Part model, mm, in its own coordinate system. A direction names the side the tool comes from. Round coordinates to 2 decimals unless told otherwise and drop trailing zeros. Loops run counter-clockwise (first coordinate to the right, second up) from the corner with the lowest first, then second, coordinate; pieces in that order, holes last. Notation, with made-up numbers: M 38,-3.75 L 57,-3.75 A21 ccw 57,34.25 Z; hole C 49,78 d6. An arc over 180 degrees is marked long. Write each question's results on one line, items separated by ' | '.
from build123d import *

# Parameters (mm, degrees)
BOSS_EXTRUDE1_DEPTH = 6.35
SKETCH9_R           = 3.175
CUT_EXTRUDE3_DEPTH  = 7.35
CIRPATTERN6_COUNT   = 3
CUT_EXTRUDE4_DEPTH  = 7.35
BOSS_EXTRUDE4_DEPTH = 6.35
CIRPATTERN7_COUNT   = 6


with BuildPart() as part:
    # Sketch1 → Boss-Extrude1 (new body)
    with BuildSketch(Plane(origin=(0, 0, 0), x_dir=(1, 0, 0), z_dir=(0, 1, 0))):
        Polygon((88.9, 0), (44.45, 76.989658396), (-44.45, 76.989658396), (-88.9, 0), (-44.45, -76.989658396), (44.45, -76.989658396), align=None)
    extrude(amount=-BOSS_EXTRUDE1_DEPTH)

    # Sketch9 → Cut-Extrude3 (cut, through all)
    with BuildSketch(Plane(origin=(0, 0, 0), x_dir=(1, 0, 0), z_dir=(0, 1, 0))):
        with Locations((-50.8, -29.329393675)):
            Circle(SKETCH9_R)
    cut_extrude3 = extrude(amount=-CUT_EXTRUDE3_DEPTH, mode=Mode.SUBTRACT)

    # CirPattern6: Cut-Extrude3 ×3 about axis
    cirpattern6_axis = Axis((0, 0, 0), (0, 1, 0))
    for i in range(1, CIRPATTERN6_COUNT):
        add(cut_extrude3.rotate(cirpattern6_axis, i * 360 / CIRPATTERN6_COUNT), mode=Mode.SUBTRACT)

    # Sketch10 → Cut-Extrude4 (cut, through all)
    with BuildSketch(Plane(origin=(0, 0, 0), x_dir=(1, 0, 0), z_dir=(0, 1, 0))):
        Polygon((57.15, 54.99261314), (48.475738686, 57.316874454), (61.175738686, 35.319829198), (66.675, 38.494829198), align=None)
    cut_extrude4 = extrude(amount=-CUT_EXTRUDE4_DEPTH, mode=Mode.SUBTRACT)

    # Sketch11 → Boss-Extrude4 (add)
    with BuildSketch(Plane(origin=(0, 0, 0), x_dir=(1, 0, 0), z_dir=(0, 1, 0))):
        Polygon((66.675, 38.494829198), (72.174261314, 41.669829198), (84.874261314, 19.672783942), (76.2, 21.997045256), align=None)
    boss_extrude4 = extrude(amount=-BOSS_EXTRUDE4_DEPTH)

    # CirPattern7: Cut-Extrude4, Boss-Extrude4 ×6 about axis
    cirpattern7_axis = Axis((0, 0, 0), (0, 1, 0))
    for i in range(1, CIRPATTERN7_COUNT):
        add(cut_extrude4.rotate(cirpattern7_axis, i * 360 / CIRPATTERN7_COUNT), mode=Mode.SUBTRACT)
        add(boss_extrude4.rotate(cirpattern7_axis, i * 360 / CIRPATTERN7_COUNT))


solid = part.part
Item 1: Wall check: L1, parallel to X at y = -4.5, z = -57.5; L2, parallel to Z at x = 50.8, y = -4.5; L3, parallel to Z at x = -50.8, y = -3.25. Give the ranges that are in metal, low to high.
Filled sheet:
L1: -63.03 to -57.82, -55.7 to -2.96, 2.96 to 55.7 | L2: -65.99 to -56.69, -53.29 to 26.15, 32.5 to 65.99 | L3: -65.99 to 26.15, 32.5 to 53.29, 56.69 to 65.99
Item 2: Band-saw the part on B-B on z = -44. Give the cut face in (x, y).
Filled sheet:
outline: M -70.83,-6.35 L 56.16,-6.35 L 56.16,0 L -70.83,0 Z
Item 3: Drop flat-ended pins along their axis: P1, Ø2, axis at y = -4.5, z = 13.5, coming from the -X side; P2, Ø3, axis at y = -4, z = 66.5, coming from the -X side; P3, Ø1, axis at y = -5.5, z = -11.5, coming from the +X side. Give the stop position or say it passes through.
Filled sheet:
P1: x = -81.68 | P2: x = -51.37 | P3: x = 82.55
Item 4: Two-plate mould, pull along X, no slides. Class faces 1 (the flat face through (-32, -3, -76.99)), 2 (the flat face through (-82.461, -3.131, -11.153)), 3 (the flat face through (-80.6, -3.13, 20.82)), 4 (the flat face through (22.18, -3.13, 73.86)): +X half, -X half, draft (parallel to the pull), parting line (faces both ways), or undercut.
Filled sheet:
face 1: draft | face 2: -X half | face 3: undercut | face 4: undercut
Item 5: Band-saw the part on D-D on z = 52.5. Give the cut face in (x, y), and give its area (3 significant figures).
Filled sheet:
outline: M -51.26,-6.35 L 65.92,-6.35 L 65.92,0 L -51.26,0 Z | area: 744 mm^2
Item 6: Band-saw the part on A-A on x = -50.8. Give the cut face in (y, z), and give its area (3 significant figures).
Filled sheet:
outline: M -6.35,-65.99 L 0,-65.99 L 0,26.15 L -6.35,26.15 Z; M -6.35,32.5 L 0,32.5 L 0,53.29 L -6.35,53.29 Z; M -6.35,56.69 L 0,56.69 L 0,65.99 L -6.35,65.99 Z | area: 776 mm^2
Item 7: Which spindle directions (+Z, -Z, +X, -X, +Y, -Y) get a long thin tool onto all of the face, cutting with end or side? Do faces 5 (the flat face through (32, -3, 76.99)), 6 (the flat face through (54.74, -3.13, -46.47)), 7 (the flat face through (32, -3, -76.99)). Say none if no direction does.
Filled sheet:
face 5: +Z, +X, +Y, -Y | face 6: +Y, -Y | face 7: +X, +Y, -Y
Item 8: Band-saw the part on C-C on y = -2.25. Count the separate pieces of the cut face and the enclosed holes in it, and give its area (3 significant figures).
Filled sheet:
separate pieces: 1 | enclosed holes: 3 | area: 20,400 mm^2
